Can you work these out from the model? Positions are in its coordinate system, mm. Give positions to 0.01 mm unless a question says otherwise; leave off trailing zeros. Loops run counter-clockwise (first coordinate to the right, second up) from the corner with the lowest first, then second, coordinate; pieces in that order, holes last. Notation, with made-up numbers: (26, 86) - (37, 86) arc R37 ccw to (37, 122) - close; hole circle Ø1 at (1, -31). An arc over 180 degrees is marked (long way). Write item = value, one per line.
from build123d import *

# Parameters (mm, degrees)
F0_W     = 6.35
F0_H     = 12.7
F1_DEPTH = 3.175
F2_DEPTH = 0.79375
F3_DEPTH = 0.79375
F5_DEPTH = 1.5875
F7_DEPTH = 1.5875


with BuildPart() as f1:
    # F0 (on Front) → F1 (new body)
    with BuildSketch(Plane.XZ):
        with Locations((-39.4517260957, 26.0147806257)):
            Rectangle(F0_W, F0_H)
    extrude(amount=F1_DEPTH)

    # F2 (add): a face of the model
    f2_faces = [f1.faces().sort_by_distance(p)[0] for p in [
        (-39.4517260957, -1.5875, 19.6647806257),
    ]]
    extrude(f2_faces, amount=F2_DEPTH)

    # F3 (add): a face of the model
    f3_faces = [f1.faces().sort_by_distance(p)[0] for p in [
        (-39.4517260957, -1.5875, 32.3647806257),
    ]]
    extrude(f3_faces, amount=F3_DEPTH)

    # F4 (on face) → F5 (join)
    with BuildSketch(Plane(origin=(-42.6267260957, 0, 0), x_dir=(0, -1, 0), z_dir=(-1, 0, 0))):
        with BuildLine():
            ThreePointArc((1.5875, 33.1585306257), (1.0262339924, 31.8035146181), (2.38125, 32.3647806257))
            ThreePointArc((2.38125, 32.3647806257), (2.1487660076, 32.9260466333), (1.5875, 33.1585306257))
        make_face()
        with BuildLine():
            ThreePointArc((2.38125, 19.6647806257), (1.0262339924, 20.2260466333), (1.5875, 18.8710306257))
            ThreePointArc((1.5875, 18.8710306257), (2.1487660076, 19.1035146181), (2.38125, 19.6647806257))
        make_face()
    extrude(amount=F5_DEPTH)

    # F6 (on face) → F7 (join)
    with BuildSketch(Plane.YZ.offset(-36.2767260957)):
        with BuildLine():
            ThreePointArc((-1.5875, 33.1585306257), (-2.1487660076, 31.8035146181), (-0.79375, 32.3647806257))
            ThreePointArc((-0.79375, 32.3647806257), (-1.0262339924, 32.9260466333), (-1.5875, 33.1585306257))
        make_face()
        with BuildLine():
            ThreePointArc((-0.79375, 19.6647806257), (-2.1487660076, 20.2260466333), (-1.5875, 18.8710306257))
            ThreePointArc((-1.5875, 18.8710306257), (-1.0262339924, 19.1035146181), (-0.79375, 19.6647806257))
        make_face()
    extrude(amount=F7_DEPTH)


solid = f1.part
Q1. Imagine slicing it at B-B, the plane y = -1. Write out the boundary of the cut face in (x, z), then the cut area to 3 significant figures.
Output:
outline = (-44.21, 19.13) - (-42.63, 19.13) - (-42.63, 18.87) - (-36.28, 18.87) - (-36.28, 19.13) - (-34.69, 19.13) - (-34.69, 20.2) - (-36.28, 20.2) - (-36.28, 31.83) - (-34.69, 31.83) - (-34.69, 32.9) - (-36.28, 32.9) - (-36.28, 33.16) - (-42.63, 33.16) - (-42.63, 32.9) - (-44.21, 32.9) - (-44.21, 31.83) - (-42.63, 31.83) - (-42.63, 20.2) - (-44.21, 20.2) - close
area = 97.5 mm2
Q2. Imagine slicing it at A-A, the plane x = -43. Write out the boundary of the cut face in (y, z).
Output:
outline = circle Ø1.59 at (-1.59, 19.66); circle Ø1.59 at (-1.59, 32.36)
Q3. We'd pull the mould along Z, two halves only. Please class faces 1 (the flat face through (-34.689, -2, 32)), 2 (the flat face through (-36.277, -2, 26)), 3 (the flat face through (-39, -2, 18.871)): released by +Z, released by -Z, zero draft, split by the parting line, or undercut.
Output:
face_1 = zero draft
face_2 = undercut
face_3 = released by -Z
Q4. Imagine slicing it at D-D, the plane y = -2.8. Write out the boundary of the cut face in (x, z).
Output:
outline = (-42.63, 18.87) - (-36.28, 18.87) - (-36.28, 33.16) - (-42.63, 33.16) - close
Q5. I need wall thicknesses on L1, parallel to X at y = -0.8, z = 26; L2, parallel to Z at x = -43.25, y = -2.25; L3, parallel to Z at x = -43.5, y = -2.05. Which ranges of each line are inside material? Lowest first, please.
Output:
L1 = -42.63 to -36.28
L2 = 19.23 to 20.1, 31.93 to 32.8
L3 = 19.02 to 20.31, 31.72 to 33.01
Q6. For pin 1 (1 mm diameter, centred on y = -2, z = 25, fed in from +X); pin 2 (1 mm diameter, centred on y = -2, z = 27, fed in from -X), each with a flat end and sliding along its axis, tell me the tip position at first contact or that it passes through.
Output:
pin_1 = -36.28
pin_2 = -42.63
Q7. Imagine slicing it at C-C, the plane z = 22.25. Write out the boundary of the cut face in (x, y) (3 decimals), then the cut area to 3 significant figures.
Output:
outline = (-42.627, -3.175) - (-36.277, -3.175) - (-36.277, 0) - (-42.627, 0) - close
area = 20.2 mm2
